from build123d import *

# Parameters (mm, degrees)
CHAFL_N1_SIZE = 0.2


with BuildPart() as part:
    # Croquis1 → Revolución1 (revolve)
    with BuildSketch(Plane(origin=(0, 0, 0), x_dir=(1, 0, 0), z_dir=(0, 1, 0))):
        Polygon((0, 0), (25, 0), (25, 1.5), (24, 1.5), (24, 1.198324022), (23.5, 1.198324022), (23.5, 1.5), (0, 1.5), align=None)
    revolve(axis=Axis((0, 0, 0), (1, 0, 0)))

    # Chaflán1
    chafl_n1_edges = [part.edges().sort_by_distance(p)[0] for p in [
        (25, 0, 1.5),
    ]]
    chamfer(chafl_n1_edges, length=CHAFL_N1_SIZE)


solid = part.part
The listing builds one solid part. Answer for the finished solid, in the listing's coordinates (mm). Round coordinates to 2 decimals unless told otherwise and drop trailing zeros. Order: outer loops, then holes, each group sorted by start corner. A loop starts at its lowest first (then second) coordinate and runs counter-clockwise, first axis right, second up. Notation, with made-up numbers: (-22, -31.5) - (15, -31.5) arc R25 cw to (15, 4.5) - close; hole circle Ø7 at (66.25, -27.75). An arc over 180 degrees is marked (long way). Write item = value, one per line. Start each with the question number.
1) Straight lines are drawn through the part: L1, parallel to X at y = -1.3, z = 0.2; L2, parallel to Y at x = 5.75, z = 0.1. For each, find the intervals that lie inside material, in ascending order.
2) Section A-A, the plane x = 11.5 is taken. Write down the section's boundary in (y, z), plus the area to 3 significant figures.
3) For a pull along X with two mould halves and no side action, classify faces 1 (the flat face through (0, 0, 0)), 2 (the cylindrical face through (24.39, 0.07, 1.5)), 3 (the cylindrical face through (23.746, 0.053, 1.197)) as released by +X, released by -X, zero draft, split by the parting line, or undercut.
Results list:
q1.L1 = 0 to 23.5, 24 to 24.98
q1.L2 = -1.5 to 1.5
q2.outline = circle Ø3 at (0, 0)
q2.area = 7.07 mm^2
q3.face_1 = released by -X
q3.face_2 = zero draft
q3.face_3 = undercut
